The listing builds one solid part. Answer for the finished solid, in the listing's coordinates (mm). Face numbers are marked on the shaded views. A direction names the side the tool comes from. Coordinates: 2 decimals unless noted, no trailing zeros. Loops run counter-clockwise (first coordinate to the right, second up) from the corner with the lowest first, then second, coordinate; pieces in that order, holes last. Notation, with made-up numbers: (32.5, -22.75) -> (74.5, -22.75) arc R15 ccw to (74.5, -17.75) -> close; hole circle Ø11 at (-35, 77). An arc over 180 degrees is marked (long way). Answer in a Markdown table with one row per item.
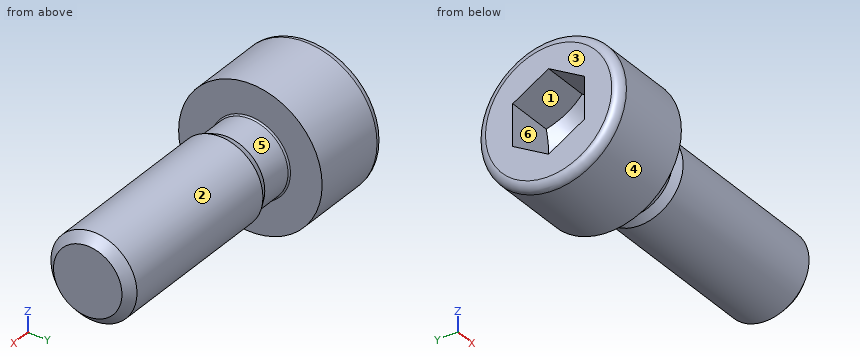
Autodesk Inventor part; units mm, degrees
ref_plane "Work Plane1" through (29, 0, 0) normal (0, -1, 0) x (1, 0, 0)
ref_plane "YZ Plane" through (0, 0, 0) normal (1, 0, 0) x (0, 1, 0)
ref_plane "XZ Plane" through (0, 0, 0) normal (0, 1, 0) x (-1, 0, 0)
sketch "Sketch1" plane through (0, 0, 0) normal (0, 0, 1) x (1, 0, 0)
  line L0 (-1.0333, 0) -> (16, 0)
  line L1 (16, 0) -> (16, 3)
  line L2 (16, 3) -> (3, 3)
  line L3 (3, 3) -> (2.3864, 2.6933)
  line L4 (2.3864, 2.6933) -> (0, 2.6933)
  line L5 (0, 2.6933) -> (0, 5)
  line L6 (0, 5) -> (-6, 5)
  line L7 (-6, 5) -> (-6, 2.8868)
  line L8 (-6, 2.8868) -> (-2.7, 2.8868)
  line L9 (-2.7, 2.8868) -> (-1.0333, 0)
  line L10 (-10.4, 0) -> (20.4, 0)
  line L11 (0, -1) -> (0, 6)
  line L12 (3, 3) -> (0, 3) construction
  dimension "d1" = 13
  dimension "d2" = 0.6136
  dimension "d3" = 6
  dimension "d4" = 3.3
  dimension "d5" = 60
  dimension "d6" = 6
  dimension "d7" = 5.3865
  dimension "d8" = 5.7735
  dimension "d9" = 10
  dimension "d26" = 16
revolve "Body" add sketch "Sketch1" angle 360 about axis through (-1.0333, 0, 0) along (1, 0, 0)
sketch "Sketch2" plane through (-6, 0, 0) normal (-1, 0, 0) x (0, 0, 1)
  circle A0 centre (0, 0) radius 2.8868
  line L0 (0, -7) -> (0, 7)
  line L1 (-7, 0) -> (7, 0)
  line L2 (2.8868, 0) -> (1.4434, -2.5)
  line L3 (1.4434, -2.5) -> (-1.4434, -2.5)
  line L4 (-1.4434, -2.5) -> (-2.8868, 0)
  line L5 (-2.8868, 0) -> (-1.4434, 2.5)
  line L6 (-1.4434, 2.5) -> (1.4434, 2.5)
  line L7 (1.4434, 2.5) -> (2.8868, 0)
extrude "Slot" add sketch "Sketch2" against normal up to next contours L7 A0 | A0 L2 | L6 L0 A0 | A0 L0 L3 | L0 L6 A0 | A0 L3 L0 | L4 A0 | A0 L5
fillet "Fillet1" radius 0.6 1 edges at (-6, -5, 0)
thread "Thread"
chamfer "Chamfer1" distance 0.6135 distance2 0.6135 1 edges at (16, -3, 0) measured on face at (16, -1.1424, 0.935)
ref_plane "Work Plane1" through (29, 0, 0) normal (0, -1, 0) x (1, 0, 0)
fillet "Fillet2" radius 0.1 1 edges at (0, -2.6933, 0)
equation "\"d1\" = GEL"
equation "\"d3\" = KOH"
equation "\"d4\" = INTI"
equation "\"d6\" = GD"
equation "\"d7\" = BDM"
equation "\"d8\" = 1.1547 * SW"
equation "\"d9\" = KOD"
equation "\"d26\" = NLG"
equation "\"d30\" = R"
equation "\"d17\" = RR"
equation "\"d13\" = GEL"
equation "\"d15\" = -0.5 * SPD + 0.5 * GD"
equation "\"d16\" = GUL"
equation "\"GD\" = NND"
equation "\"NLG\" = 16"
equation "\"GEL\" = 13"
equation "\"KOD\" = 10"
equation "\"KOH\" = NND"
equation "\"INTI\" = 3.3"
equation "\"GAL\" = 0.61345 * PTC"
equation "\"GUL\" = 0.61345 * PTC"
equation "\"BDM\" = 5.3865"
equation "\"SW\" = 5"
equation "\"RR\" = 0.6"
equation "\"SPD\" = NND - 1.2269 * PTC"
equation "\"R\" = 0.1"
equation "\"PHH\" = 0.5"
equation "\"GD1\" = THREADDIA - 1.2269 * PTC"
equation "\"THREADDIA\" = 6"
equation "\"FAWI\" = 45deg"
equation "\"PTC\" = 1"
equation "\"NND\" = 6"
equation "\"TOA\" = 30deg"
equation "\"E0\" = 1.155 * SW"
properties part number "CSN 02 1143 - M6 x 16" material "Steel, Mild"
Item 1: Determine the mould class of the marked faces 1, 2 and 3 for opening direction Y: +Y half, -Y half, draft (parallel to the pull), parting line (faces both ways), or undercut.
Findings below:
| item | result |
|---|---|
| face 1 | undercut |
| face 2 | parting line |
| face 3 | draft |
Item 2: Flat-ended cylindrical pins translate along their axes: pin 1 Ø5 at (x, z) = (0.5, 1) entering from +Y; pin 2 Ø2 at (x, z) = (3.5, -2.5) entering from +Y; pin 3 Ø2 at (x, z) = (5.5, 3.5) entering from -Y; pin 4 Ø1.5 at (x, z) = (6, 0) entering from +Y. Find the tip coordinate at first contact, or state that the pin passes through.
Findings below:
| item | result |
|---|---|
| pin 1 | stops at y = 5 |
| pin 2 | stops at y = 2.6 |
| pin 3 | stops at y = -1.66 |
| pin 4 | stops at y = 3 |
Item 3: A cutting plane is placed at A-A, the plane x = 1. Determine the outline of the cut face in (y, z).
Findings below:
| item | result |
|---|---|
| outline | circle Ø5.39 at (0, 0) |
Item 4: Find the intervals of material crossed by probe 1 along X at (y, z) = (-3, 0.5); probe 2 along Y at (x, z) = (-3, -2.75); probe 3 along Y at (x, z) = (-1.5, -0.25), in increasing order.
Findings below:
| item | result |
|---|---|
| probe 1 | x = -6 to 0 |
| probe 2 | y = -4.18 to -0.24, 0.24 to 4.18 |
| probe 3 | y = -4.99 to -0.77, 0.77 to 4.99 |
Item 5: A tool of negligible diameter and unlimited length cuts with its end or side. For the marked faces 4, 5 and 6, from which of +Z, -Z, +X, -X, +Y, -Y can it reach the whole face along a straight path? Write none if from no direction.
Findings below:
| item | result |
|---|---|
| face 4 | +X, -X |
| face 5 | none |
| face 6 | -X |
